from build123d import *

# Parameters (mm, degrees)
F0_W     = 60
F0_H     = 50
F1_DEPTH = 10
F2_R     = 5
F3_T     = -1.5


with BuildPart() as f1:
    # F0 (on Front) → F1 (new body)
    with BuildSketch(Plane.XZ):
        with Locations((-30, 25)):
            Rectangle(F0_W, F0_H)
    extrude(amount=F1_DEPTH)

    # F2
    f2_edges = [f1.edges().sort_by_distance(p)[0] for p in [
        (-60, -5, 50),
        (-30, -10, 50),
        (-60, -10, 25),
        (-30, -10, 0),
        (0, -10, 25),
        (0, -5, 50),
        (-60, -5, 0),
        (0, -5, 0),
    ]]
    fillet(f2_edges, radius=F2_R)

    # F3
    f3_openings = [f1.faces().sort_by_distance(p)[0] for p in [
        (-30, 0, 25),
    ]]
    offset(amount=F3_T, openings=f3_openings)


solid = f1.part
Check sheet for the modelled part. Datum: model origin and axes. Units: mm. A direction names the side the tool comes from. Round coordinates to 2 decimals unless told otherwise and drop trailing zeros. Loops run counter-clockwise (first coordinate to the right, second up) from the corner with the lowest first, then second, coordinate; pieces in that order, holes last. Notation, with made-up numbers: (85.5, -6) -> (96.5, -6) arc R18 cw to (96.5, 28) -> close; hole circle Ø9 at (-38, 66). An arc over 180 degrees is marked (long way). Put each result on its own line as item: value. Start each with the question number.
1. Section check A-A (y = -1.75). Enter the section's corners in (x, z).
2. Section check D-D (y = -6.75). Enter the section's corners in (x, z).
3. Section check C-C (z = 16). Enter the section's corners in (x, y).
4. Draft check along X on faces 3 (the face through (-57.5, -2.54, 2.55)), 4 (the face through (-1, -3, 48)), 5 (the face through (-30, 0, 49)), 6 (the face through (-59, -3, 48)). Enter one of: +X half, -X half, draft (parallel to the pull), parting line (faces both ways), or undercut.
5. Gauge pin test, flat ends, axial feed: pin 1 (1 mm diameter, centred on y = -7, z = 35.5, fed in from +X); pin 2 (20 mm diameter, centred on x = -32, z = 20, fed in from +Y). Record the tip position at first contact, or that the pin passes through.
6. Scan lines: probe 1 along X at (y, z) = (-1, 39.5); probe 2 along Z at (x, y) = (-33, -2); probe 3 along Y at (x, z) = (-22, 18). Record each from-to range of solid material in increasing order.
7. Access from +Z, -Z, +X, -X, +Y, -Y to the whole of each face (thin tool, end or side, straight path). Record for faces 1 (the face through (-30, -2, 48.5)), 2 (the face through (-1, -8, 25)).
8. Section check B-B (x = -41). Enter the section's corners in (y, z).
Findings:
1. outline: (-60, 5) arc R5 ccw to (-55, 0) -> (-5, 0) arc R5 ccw to (0, 5) -> (0, 45) arc R5 ccw to (-5, 50) -> (-55, 50) arc R5 ccw to (-60, 45) -> close; hole (-58.5, 5) arc R3.5 ccw to (-55, 1.5) -> (-5, 1.5) arc R3.5 ccw to (-1.5, 5) -> (-1.5, 45) arc R3.5 ccw to (-5, 48.5) -> (-55, 48.5) arc R3.5 ccw to (-58.5, 45) -> close
2. outline: (-59.68, 5) arc R4.68 ccw to (-55, 0.32) -> (-5, 0.32) arc R4.68 ccw to (-0.32, 5) -> (-0.32, 45) arc R4.68 ccw to (-5, 49.68) -> (-55, 49.68) arc R4.68 ccw to (-59.68, 45) -> close; hole (-58.03, 5) arc R3.03 ccw to (-55, 1.97) -> (-5, 1.97) arc R3.03 ccw to (-1.97, 5) -> (-1.97, 45) arc R3.03 ccw to (-5, 48.03) -> (-55, 48.03) arc R3.03 ccw to (-58.03, 45) -> close
3. outline: (-60, -5) arc R5 ccw to (-55, -10) -> (-5, -10) arc R5 ccw to (0, -5) -> (0, 0) -> (-1.5, 0) -> (-1.5, -5) arc R3.5 cw to (-5, -8.5) -> (-55, -8.5) arc R3.5 cw to (-58.5, -5) -> (-58.5, 0) -> (-60, 0) -> close
4. face 3: undercut
4. face 4: +X half
4. face 5: draft
4. face 6: -X half
5. pin 1: stops at x = -0.23
5. pin 2: stops at y = -8.5
6. probe 1: x = -60 to -58.5, -1.5 to 0
6. probe 2: z = 0 to 1.5, 48.5 to 50
6. probe 3: y = -10 to -8.5
7. face 1: +Y
7. face 2: +Z, -Z, +X, -Y
8. outline: (-10, 5) arc R5 ccw to (-5, 0) -> (0, 0) -> (0, 1.5) -> (-5, 1.5) arc R3.5 cw to (-8.5, 5) -> (-8.5, 45) arc R3.5 cw to (-5, 48.5) -> (0, 48.5) -> (0, 50) -> (-5, 50) arc R5 ccw to (-10, 45) -> close
